Work out the finished part from the listing and answer in its coordinate system (mm). Round coordinates to 2 decimals unless told otherwise and drop trailing zeros. Loops run counter-clockwise (first coordinate to the right, second up) from the corner with the lowest first, then second, coordinate; pieces in that order, holes last. Notation, with made-up numbers: (-31, 43.25) - (-7, 43.25) arc R11 ccw to (-7, 54.25) - close; hole circle Ø8 at (65, 38.25). An arc over 180 degrees is marked (long way). Answer as CSV lines item,"result". Start each with the question number.
Q1. The mould has two halves that part along Y. Classify faces 1 (the face through (-48.26, 185.98, -7.1)), 2 (the face through (-28.99, 165.25, -105.19)), 3 (the face through (-38, 176, 0)): +Y half, -Y half, draft (parallel to the pull), parting line (faces both ways), or undercut.
Q2. Each of these flat-tipped pins is pushed along its axis until it touches: pin 1 Ø8 at (y, z) = (182, -73) entering from +X; pin 2 Ø4 at (x, y) = (-21, 155) entering from -Z; pin 3 Ø3 at (y, z) = (110, -164) entering from +X; pin 4 Ø12 at (x, y) = (6, 119.5) entering from +Z. Where does it stop, or does it pass through?
Q3. Section C-C on x = -43 is taken. Write down the section's boundary in (y, z), then the cut area to 3 significant figures.
Q4. Section A-A on z = -43.5 is taken. Write down the section's boundary in (x, y), then the cut area to 3 significant figures.
Q5. Straight lines are drawn through the part: L1, parallel to X at y = 191, z = -157.5; L2, parallel to Y at x = 1.5, z = -183.5; L3, parallel to Y at x = 3.5, z = -112.5. For each, find the intervals that lie inside material, in ascending order. Write a range as [from, to].
Q6. Section B-B on y = 100 is taken. Write down the section's boundary in (x, z), then the cut area to 3 significant figures.
Autodesk Inventor part; units mm, degrees
ref_plane "YZ Plane" through (0, 0, 0) normal (1, 0, 0) x (0, 1, 0)
ref_plane "XZ Plane" through (0, 0, 0) normal (0, 1, 0) x (-1, 0, 0)
ref_plane "XY Plane" through (0, 0, 0) normal (0, 0, 1) x (1, 0, 0)
sketch "Sketch1" plane through (0, 0, 0) normal (0, 0, 1) x (1, 0, 0)
  line L0 (17.2421, 103.0289) -> (10.8921, 114.0275)
  arc A0 (-38.1, 178.1746) -> (-35.7188, 175.7934) centre (-35.7188, 178.1746) ccw construction
  line L1 (-57.8926, 195.9643) -> (-60.8346, 198.1519) construction
  line L2 (-54.5271, 197.4183) -> (-57.8926, 195.9643) construction
  line L3 (-60.8346, 198.1519) -> (-60.4111, 201.7935) construction
  circle A1 centre (-57.4691, 199.6059) radius 4.7625 construction
  line L4 (26.0216, 87.8223) -> (10.8921, 114.0275)
  arc A2 (10.8921, 114.0275) -> (-77.4031, 211.1891) centre (-275.2793, -57.3297) ccw
  line L5 (24.6468, 87.0285) -> (9.5236, 113.2227)
  arc A3 (9.5236, 113.2227) -> (-78.349, 209.9142) centre (-275.2793, -57.3297) ccw
  line L6 (26.0216, 87.8223) -> (24.6468, 87.0285)
  line L7 (-77.4031, 211.1891) -> (-78.349, 209.9142)
  arc A4 (8.2879, 112.4961) -> (-75.5859, 206.0593) centre (-275.2793, -57.3297) ccw construction
  line L8 (8.2879, 112.4961) -> (24.1221, 85.0704) construction
  point P0 (0, 0)
  dimension "d0" = 1.5875
  dimension "d26" = 1.4334
extrude "main extrusion" add sketch "Sketch1" against normal blind 213.36
sketch "Sketch2" plane through (9.5236, 113.2227, -213.36) normal (-0.866, -0.5, 0) x (0, 0, 1)
  line L0 (213.36, -30.2465) -> (213.36, 0.0127)
  line L1 (213.36, -1.1707) -> (194.31, -1.1707)
  line L2 (194.31, -1.1707) -> (194.31, 24.2293)
  line L3 (194.31, 24.2293) -> (213.36, 24.2293)
  line L4 (213.36, 24.2293) -> (213.36, -1.1707)
  line L5 (194.31, -1.1707) -> (0, -1.1707) construction
  line L6 (213.36, 0.0127) -> (0, 0.0127) construction
  line L7 (0, -1.1707) -> (19.05, -1.1707)
  line L8 (19.05, -1.1707) -> (19.05, 24.2293)
  line L9 (19.05, 24.2293) -> (0, 24.2293)
  line L10 (0, 24.2293) -> (0, -1.1707)
  point P0 (213.36, -93.292)
  dimension "d3" = 19.05
  dimension "d4" = 25.4
  dimension "d5" = 19.05
  dimension "d6" = 25.4
extrude "square side cuts" cut sketch "Sketch2" along normal blind 2.54 and the other way blind 2.54
fillet "square cut fillets" radius 2.54 4 edges at (-3.004, 133.9675, -213.36) (-3.004, 133.9675, 0) (10.7964, 112.6057, 0) (10.7964, 112.6057, -213.36)
ref_plane "Work Plane1" through (0, 0, -5.08) normal (0, 0, 1) x (1, 0, 0)
ref_plane "Work Plane2" through (-50.8851, 191.5138, -213.36) normal (-0.8031, 0.5959, 0) x (0, 0, 1)
hole "Hole1" at (-48.3442, 184.9538, -5.08) direction (0.6836, 0.7298, 0) diameter 4.2418 depth 12.7
ref_plane "Work Plane3" through (0, 0, -8.89) normal (0, 0, 1) x (1, 0, 0)
ref_plane "Work Plane4" through (-26.407, 173.352, -213.36) normal (-0.8031, 0.5959, 0) x (0, 0, 1)
hole "Hole2" at (-26.8136, 162.8194, -8.89) direction (0.7485, 0.6632, 0) diameter 4.2418 depth 12.7
ref_plane "Work Plane5" through (0, 0, -25.4) normal (0, 0, 1) x (1, 0, 0)
ref_plane "Work Plane6" through (-3.9687, 156.7036, -213.36) normal (-0.8031, 0.5959, 0) x (0, 0, 1)
hole "Hole5" at (-8.6418, 140.4208, -25.4) direction (0.8032, 0.5957, 0) diameter 4.2418 depth 12.7
ref_plane "Work Plane7" through (0, 0, -208.28) normal (0, 0, -1) x (-1, 0, 0)
ref_plane "Work Plane8" through (-50.8851, 191.5138, -213.36) normal (-0.8031, 0.5959, 0) x (0, 0, 1)
hole "Hole6" at (-48.3442, 184.9538, -208.28) direction (0.6836, 0.7298, 0) diameter 4.2418 depth 12.7
ref_plane "Work Plane9" through (0, 0, -204.47) normal (0, 0, -1) x (-1, 0, 0)
ref_plane "Work Plane10" through (-26.407, 173.352, -213.36) normal (-0.8031, 0.5959, 0) x (0, 0, 1)
hole "Hole7" at (-26.8136, 162.8194, -204.47) direction (0.7485, 0.6632, 0) diameter 4.2418 depth 12.7
ref_plane "Work Plane11" through (0, 0, -187.96) normal (0, 0, -1) x (-1, 0, 0)
ref_plane "Work Plane12" through (-3.9687, 156.7036, -213.36) normal (-0.8031, 0.5959, 0) x (0, 0, 1)
hole "Hole8" at (-8.6418, 140.4208, -187.96) direction (0.8032, 0.5957, 0) diameter 4.2418 depth 12.7
sketch "Sketch4" plane through (24.6468, 87.0285, -213.36) normal (-0.866, -0.5, 0) x (0, 0, 1)
  circle A0 centre (26.67, 23.9091) radius 2.1209
  circle A1 centre (186.69, 23.9091) radius 2.1209
  arc A2 (22.0345, 23.9091) -> (26.2255, 23.9091) centre (24.13, 23.9091) ccw construction
  line L0 (24.13, 23.9091) -> (26.67, 23.9091) construction
  arc A3 (187.1345, 23.9091) -> (191.3255, 23.9091) centre (189.23, 23.9091) ccw construction
  line L1 (189.23, 23.9091) -> (186.69, 23.9091) construction
  point P0 (213.36, -63.0455)
  dimension "d102" = 4.2418
  dimension "d105" = 4.2418
  dimension "d109" = 2.54
  dimension "d110" = 2.54
extrude "top screw holes" cut sketch "Sketch4" against normal blind 1.5875
properties part number "! Intake polycarb" material "Polycarbonate, Clear"
Findings:
1,face 1,"undercut"
1,face 2,"-Y half"
1,face 3,"draft"
2,pin 1,"stops at x = -38.9"
2,pin 2,"stops at z = -213.36"
2,pin 3,"stops at x = 14.08"
2,pin 4,"stops at z = -19.05"
3,outline,"(179.84, -213.36) - (182.05, -213.36) - (182.05, 0) - (179.84, 0) - close"
3,area,"473 mm^2"
4,outline,"(-78.35, 209.91) arc R331.97 cw to (9.52, 113.22) - (24.65, 87.03) - (26.02, 87.82) - (17.24, 103.03) - (10.89, 114.03) arc R333.55 ccw to (-77.4, 211.19) - close"
4,area,"257 mm^2"
5,L1,"x = [-54.98, -52.59]"
5,L2,"y = [125.96, 128.82]"
5,L3,"y = [122.9, 125.81]"
6,outline,"(17.16, -213.36) - (18.99, -213.36) - (18.99, 0) - (17.16, 0) - close"
6,area,"391 mm^2"
